from build123d import *

# Parameters (mm, degrees)
SKETCH1_R           = 30
BOSS_EXTRUDE1_DEPTH = 30


with BuildPart() as part:
    # Sketch1 → Boss-Extrude1 (new body)
    with BuildSketch(Plane.XY):
        with BuildLine():
            ThreePointArc((-25.980762114, 15), (-15, 25.980762114), (0, 30))
            Line((0, 30), (0, 38))
            ThreePointArc((0, 38), (-7.295122504, 37.293178836), (-14.318858324, 35.199009877))
            Line((-14.318858324, 35.199009877), (-25.980762114, 15))
        make_face()
        with BuildLine():
            ThreePointArc((-25.980762114, -15), (-30, 0), (-25.980762114, 15))
            Line((-25.980762114, 15), (-32.908965344, 19))
            ThreePointArc((-32.908965344, 19), (-35.944401511, 12.328828006), (-37.642665903, 5.199009877))
            Line((-37.642665903, 5.199009877), (-25.980762114, -15))
        make_face()
        with BuildLine():
            ThreePointArc((0, -30), (-15, -25.980762114), (-25.980762114, -15))
            Line((-25.980762114, -15), (-32.908965344, -19))
            ThreePointArc((-32.908965344, -19), (-28.649279008, -24.96435083), (-23.323807579, -30))
            Line((-23.323807579, -30), (0, -30))
        make_face()
        with BuildLine():
            Line((14.318858324, -35.199009877), (25.980762114, -15))
            ThreePointArc((25.980762114, -15), (15, -25.980762114), (0, -30))
            Line((0, -30), (0, -38))
            ThreePointArc((0, -38), (7.295122504, -37.293178836), (14.318858324, -35.199009877))
        make_face()
        with BuildLine():
            Line((37.642665903, -5.199009877), (25.980762114, 15))
            ThreePointArc((25.980762114, 15), (28.977774789, 7.764571353), (30, 0))
            ThreePointArc((30, 0), (28.977774789, -7.764571353), (25.980762114, -15))
            Line((25.980762114, -15), (32.908965344, -19))
            ThreePointArc((32.908965344, -19), (35.944401511, -12.328828006), (37.642665903, -5.199009877))
        make_face()
        with BuildLine():
            Line((8.246211251, 30), (0, 30))
            ThreePointArc((0, 30), (15, 25.980762114), (25.980762114, 15))
            Line((25.980762114, 15), (32.908965344, 19))
            ThreePointArc((32.908965344, 19), (28.649279008, 24.96435083), (23.323807579, 30))
            Line((23.323807579, 30), (8.246211251, 30))
        make_face()
        Circle(SKETCH1_R)
    extrude(amount=BOSS_EXTRUDE1_DEPTH)


solid = part.part
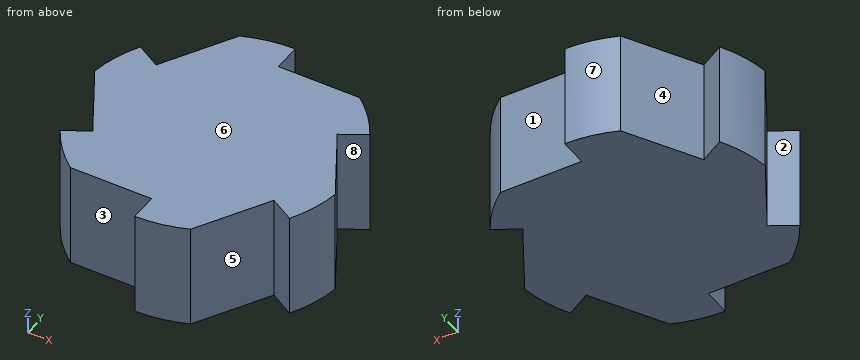
Work out the finished part from the listing and answer in its coordinate system (mm). Face numbers are marked on the shaded views. A direction names the side the tool comes from. Round coordinates to 2 decimals unless told otherwise and drop trailing zeros. Loops run counter-clockwise (first coordinate to the right, second up) from the corner with the lowest first, then second, coordinate; pieces in that order, holes last. Notation, with made-up numbers: (67, 66) -> (125, 66) arc R13 ccw to (125, 72) -> close; hole circle Ø4 at (15, -25.75). An arc over 180 degrees is marked (long way). Use one line per item in the form item = value.
(1) Find section B-B on z = 27.25. Give the vertices of the cut face in (x, y), then the cut area to 3 significant figures.
Answer list:
outline = (-37.64, 5.2) -> (-25.98, -15) -> (-32.91, -19) arc R38 ccw to (-23.32, -30) -> (0, -30) -> (0, -38) arc R38 ccw to (14.32, -35.2) -> (25.98, -15) -> (32.91, -19) arc R38 ccw to (37.64, -5.2) -> (25.98, 15) -> (32.91, 19) arc R38 ccw to (23.32, 30) -> (0, 30) -> (0, 38) arc R38 ccw to (-14.32, 35.2) -> (-25.98, 15) -> (-32.91, 19) arc R38 ccw to start
area = 3,770 mm2
(2) Find section D-D on y = 28. Give the vertices of the cut face in (x, z), then the cut area to 3 significant figures.
Answer list:
outline = (-18.48, 0) -> (25.69, 0) -> (25.69, 30) -> (-18.48, 30) -> close
area = 1,320 mm2
(3) Find section C-C on x = 27. Give the vertices of the cut face in (y, z), then the cut area to 3 significant figures.
Answer list:
outline = (-15.59, 0) -> (13.23, 0) -> (13.23, 30) -> (-15.59, 30) -> close; (15.59, 0) -> (26.74, 0) -> (26.74, 30) -> (15.59, 30) -> close
area = 1,200 mm2
(4) For a pull along Y with two mould halves and no side action, classify the marked faces 6, 7 and 8 as released by +Y, released by -Y, zero draft, split by the parting line, or undercut.
Answer list:
face_6 = zero draft
face_7 = released by +Y
face_8 = undercut
(5) Straight lines are drawn through the part: line 1 (Y direction, x = 29, z = 9.75); line 2 (X direction, y = 18, z = 12.5); line 3 (X direction, y = 16.5, z = 3.75). For each, find the intervals that lie inside material, in ascending order.
Answer list:
line_1 = -16.74 to 9.77, 16.74 to 24.56
line_2 = -33.47 to -31.18, -24.25 to 31.18
line_3 = -34.23 to -28.58, -25.11 to 28.58
(6) A tool of negligible diameter and unlimited length cuts with its end or side. For the marked faces 1, 2, 3, 4 and 5, from which of +Z, -Z, +X, -X, +Y, -Y can it reach the whole face along a straight path? Write none if from no direction.
Answer list:
face_1 = +Z, -Z, +X, +Y
face_2 = +Z, -Z, -X
face_3 = +Z, -Z, -X, -Y
face_4 = +Z, -Z, +Y
face_5 = +Z, -Z, -Y
(7) Flat-ended cylindrical pins translate along their axes: P1, Ø5, axis at x = -0.5, z = 19, coming from the +Y side; P2, Ø6, axis at x = -8.5, z = 17.5, coming from the +Y side; P3, Ø4, axis at y = 33.5, z = 20, coming from the +X side; P4, Ø2, axis at x = -17, z = 15.5, coming from the +Y side. Find the tip coordinate at first contact, or state that the pin passes through.
Answer list:
P1 = 38
P2 = 37.6
P3 = 0
P4 = 32.29
(8) Find section A-A on y = 17.5. Give the vertices of the cut face in (x, z).
Answer list:
outline = (-33.73, 0) -> (-30.31, 0) -> (-30.31, 30) -> (-33.73, 30) -> close; (-24.54, 0) -> (30.31, 0) -> (30.31, 30) -> (-24.54, 30) -> close
